Geometry check sheet. Reference: the model listing, model coordinates, mm. A direction names the side the tool comes from. Round coordinates to 2 decimals unless told otherwise and drop trailing zeros. Order: outer loops, then holes, each group sorted by start corner. A loop starts at its lowest first (then second) coordinate and runs counter-clockwise, first axis right, second up. Notation, with made-up numbers: (66, 85.25) - (94, 85.25) arc R27 cw to (94, 109.25) - close; hole circle Ø5 at (40, 59.5). An arc over 180 degrees is marked (long way). Use a Markdown table: item, result. Add a question column.
(1) Section check D-D on x = -31. Give the number of separate pieces and of enclosed holes in the cut face, then the cut area to 3 significant figures.
(2) Section check B-B on x = -28.7. Record the boundary of the cut face in (y, z), then the cut area to 3 significant figures.
(3) Section check A-A on y = 133.5. Record the boundary of the cut face in (x, z), then the cut area to 3 significant figures.
(4) Mould release check, pull along X, two halves, no side actions. Record for faces 1 (the face through (-32.5, 125.56, 48.07)), 2 (the face through (-32.4, 129.6, 41)), 3 (the face through (-28, 132, 54)): released by +X, released by -X, zero draft, split by the parting line, or undercut.
(5) Access from +Z, -Z, +X, -X, +Y, -Y to the whole of each face (thin tool, end or side, straight path). Record for faces 4 (the face through (-31, 141, 60)), 5 (the face through (-29.7, 138, 70.7)), 6 (the face through (-32.4, 129.6, 39)), 7 (the face through (-32.5, 130.94, 49.43)).
(6) Section check C-C on y = 124.5. Record the boundary of the cut face in (x, z).
(7) Gauge pin test, flat ends, axial feed: P1, Ø3, axis at x = -31, y = 131.5, coming from the -Z side; P2, Ø3.5, axis at x = -31, z = 48, coming from the +Y side; P3, Ø0.9, axis at x = -31, y = 131, coming from the -Z side. Record the tip position at first contact, or that the pin passes through.
(8) Thickness scan on line 1 along Z through (x, y) = (-30.75, 140); line 2 along Z through (x, y) = (-31, 133.5); line 3 along X through (y, z) = (131, 33.25). Record the ranges inside material, lowest first. Write a range as [from, to].
```python
from build123d import *

# Parameters (mm, degrees)
CYLINDER1866_R               = 3
CYLINDER1866_DEPTH           = 3
CYLINDER1865_R               = 3
CYLINDER1865_DEPTH           = 3
CYLINDER1867_R               = 3
CYLINDER1867_DEPTH           = 3
CYLINDER1868_R               = 3
CYLINDER1868_DEPTH           = 3
CYLINDER1854_R               = 1.5
CYLINDER1854_DEPTH           = 50
CYLINDER1855_R               = 1.5
CYLINDER1855_DEPTH           = 50
CYLINDER1856_R               = 1.5
CYLINDER1856_DEPTH           = 50
CYLINDER1853_R               = 1.5
CYLINDER1853_DEPTH           = 50
CYLINDER1851_R               = 1.5
CYLINDER1851_DEPTH           = 50
CYLINDER1851_PLACEMENT_ANGLE = 45
BOX771_W                     = 6
BOX771_H                     = 8
BOX771_DEPTH                 = 2
BOX772_W                     = 49
BOX772_H                     = 19
BOX772_DEPTH                 = 6


with BuildPart() as obj1:
    # Cylinder1866 → Cylinder1866 (new body)
    with BuildSketch(Plane(origin=(-31, 150, 72), x_dir=(1, 0, 0), z_dir=(0, -1, 0))):
        Circle(CYLINDER1866_R)
    extrude(amount=CYLINDER1866_DEPTH)


with BuildPart() as obj2:
    # Cylinder1865 → Cylinder1865 (new body)
    with BuildSketch(Plane(origin=(31, 150, 48), x_dir=(1, 0, 0), z_dir=(0, -1, 0))):
        Circle(CYLINDER1865_R)
    extrude(amount=CYLINDER1865_DEPTH)


with BuildPart() as obj3:
    # Cylinder1867 → Cylinder1867 (new body)
    with BuildSketch(Plane(origin=(31, 150, 72), x_dir=(1, 0, 0), z_dir=(0, -1, 0))):
        Circle(CYLINDER1867_R)
    extrude(amount=CYLINDER1867_DEPTH)


with BuildPart() as compound933:
    # Cylinder1868 → Cylinder1868 (new body)
    with BuildSketch(Plane(origin=(-31, 150, 48), x_dir=(1, 0, 0), z_dir=(0, -1, 0))):
        Circle(CYLINDER1868_R)
    extrude(amount=CYLINDER1868_DEPTH)

    # Compound933: union obj1, obj2, obj3
    add(obj1.part)
    add(obj2.part)
    add(obj3.part)


with BuildPart() as compound933_1:
    # Compound933 placement: moved
    add(compound933.part.moved(Location((0, -9, 0))))


with BuildPart() as obj4:
    # Cylinder1854 → Cylinder1854 (new body)
    with BuildSketch(Plane(origin=(-31, 150, 72), x_dir=(1, 0, 0), z_dir=(0, -1, 0))):
        Circle(CYLINDER1854_R)
    extrude(amount=CYLINDER1854_DEPTH)


with BuildPart() as obj5:
    # Cylinder1855 → Cylinder1855 (new body)
    with BuildSketch(Plane(origin=(31, 150, 48), x_dir=(1, 0, 0), z_dir=(0, -1, 0))):
        Circle(CYLINDER1855_R)
    extrude(amount=CYLINDER1855_DEPTH)


with BuildPart() as obj6:
    # Cylinder1856 → Cylinder1856 (new body)
    with BuildSketch(Plane(origin=(31, 150, 72), x_dir=(1, 0, 0), z_dir=(0, -1, 0))):
        Circle(CYLINDER1856_R)
    extrude(amount=CYLINDER1856_DEPTH)


with BuildPart() as compound930:
    # Cylinder1853 → Cylinder1853 (new body)
    with BuildSketch(Plane(origin=(-31, 150, 48), x_dir=(1, 0, 0), z_dir=(0, -1, 0))):
        Circle(CYLINDER1853_R)
    extrude(amount=CYLINDER1853_DEPTH)

    # Compound930: union obj4, obj5, obj6
    add(obj4.part)
    add(obj5.part)
    add(obj6.part)


with BuildPart() as compound927:
    # Cylinder1851 → Cylinder1851 (new body)
    with BuildSketch(Plane.XY):
        Circle(CYLINDER1851_R)
    extrude(amount=CYLINDER1851_DEPTH)


with BuildPart() as compound927_1:
    # Cylinder1851 placement: moved
    add(compound927.part.moved(Location((-31, 92, 0))).rotate(Axis((-31, 92, 0), (0, 0, 1)), CYLINDER1851_PLACEMENT_ANGLE))


with BuildPart() as compound926:
    # Box771 → Box771 (new body)
    with BuildSketch(Plane(origin=(-27, 89, 39), x_dir=(0, 1, 0), z_dir=(0, 0, 1))):
        with Locations((3, 4)):
            Rectangle(BOX771_W, BOX771_H)
    extrude(amount=BOX771_DEPTH)


with BuildPart() as cut579:
    # Box772 → Box772 (new body)
    with BuildSketch(Plane(origin=(-34, 83, 78), x_dir=(0, 0, -1), z_dir=(1, 0, 0))):
        with Locations((24.5, 9.5)):
            Rectangle(BOX772_W, BOX772_H)
    extrude(amount=BOX772_DEPTH)

    # Cut574: cut Compound926
    add(compound926.part, mode=Mode.SUBTRACT)

    # Cut575: cut Compound927
    add(compound927_1.part, mode=Mode.SUBTRACT)


with BuildPart() as cut579_1:
    # Cut575 placement: moved
    add(cut579.part.moved(Location((0, 39, 0))))

    # Cut578: cut Compound930
    add(compound930.part, mode=Mode.SUBTRACT)

    # Cut579: cut Compound933
    add(compound933_1.part, mode=Mode.SUBTRACT)


solid = cut579_1.part
```
Check sheet entries:
| question | item | result |
|---|---|---|
| 1 | separate pieces | 4 |
| 1 | enclosed holes | 0 |
| 1 | area | 739 mm2 |
| 2 | outline | (122, 29) - (141, 29) - (141, 46.07) - (138, 46.07) - (138, 49.93) - (141, 49.93) - (141, 70.07) - (138, 70.07) - (138, 73.93) - (141, 73.93) - (141, 78) - (122, 78) - close; hole (128, 39) - (134, 39) - (134, 41) - (128, 41) - close |
| 2 | area | 896 mm2 |
| 3 | outline | (-34, 29) - (-28, 29) - (-28, 39) - (-34, 39) - close; (-34, 41) - (-28, 41) - (-28, 78) - (-34, 78) - close; hole circle Ø3 at (-31, 48); hole circle Ø3 at (-31, 72) |
| 3 | area | 268 mm2 |
| 4 | face 1 | undercut |
| 4 | face 2 | zero draft |
| 4 | face 3 | released by +X |
| 5 | face 4 | +Z, -Z, +X, -X, +Y |
| 5 | face 5 | +Y |
| 5 | face 6 | +X, -X |
| 5 | face 7 | -Z |
| 6 | outline | (-34, 29) - (-28, 29) - (-28, 78) - (-34, 78) - close; hole circle Ø3 at (-31, 48); hole circle Ø3 at (-31, 72) |
| 7 | P1 | stops at z = 29 |
| 7 | P2 | stops at y = 138 |
| 7 | P3 | stops at z = 50 |
| 8 | line 1 | z = [29, 45.01], [50.99, 69.01], [74.99, 78] |
| 8 | line 2 | z = [29, 39], [41, 46.5], [49.5, 70.5], [73.5, 78] |
| 8 | line 3 | x = [-34, -32.5], [-29.5, -28] |
